```python
from build123d import *

# Parameters (mm, degrees)
F0_W        = 39
F0_H        = 39
F0_R        = 0.975
F1_DEPTH    = 9
F2_T1_DEPTH = 62
F4_DEPTH    = 21
F5_DEPTH    = 21
F6_DEPTH    = 5.5
F7_DEPTH    = 1.5
F8_DEPTH    = 2.5
F9_DEPTH    = 1.5
F10_R       = 1.25
F11_DEPTH   = 2.5
F12_DEPTH   = 5
F13_DEPTH   = 1


# Not quite as in the source:
# - a fillet or chamfer that OpenCascade refuses, or shapes differently, is made with other operations: its cross-section is extruded or revolved along the edge and cut away or added


with BuildPart() as f1:
    # F0 (on Top) → F1 (new body)
    with BuildSketch(Plane.XY):
        Polygon((-2.625, 21), (-21, 21), (-21, -21), (-2.625, -21), (2.625, -21), (21, -21), (21, 21), (2.625, 21), align=None)
        Rectangle(F0_W, F0_H, mode=Mode.SUBTRACT)
        Rectangle(F0_W, F0_H)
        with BuildLine():
            ThreePointArc((16, 4.25), (16.6, 4.85), (17.2, 4.25))
            Line((17.2, 4.25), (17.2, -4.25))
            ThreePointArc((17.2, -4.25), (16.6, -4.85), (16, -4.25))
            Line((16, -4.25), (16, -6.5))
            ThreePointArc((16, -6.5), (16.6, -5.9), (17.2, -6.5))
            Line((17.2, -6.5), (17.2, -15.7))
            ThreePointArc((17.2, -15.7), (18.2606601718, -18.2606601718), (15.7, -17.2))
            Line((15.7, -17.2), (6.5, -17.2))
            ThreePointArc((6.5, -17.2), (5.9, -16.6), (6.5, -16))
            Line((6.5, -16), (4.25, -16))
            ThreePointArc((4.25, -16), (4.85, -16.6), (4.25, -17.2))
            Line((4.25, -17.2), (-4.25, -17.2))
            ThreePointArc((-4.25, -17.2), (-4.85, -16.6), (-4.25, -16))
            Line((-4.25, -16), (-6.5, -16))
            ThreePointArc((-6.5, -16), (-5.9, -16.6), (-6.5, -17.2))
            Line((-6.5, -17.2), (-15.7, -17.2))
            ThreePointArc((-15.7, -17.2), (-18.2606601718, -18.2606601718), (-17.2, -15.7))
            Line((-17.2, -15.7), (-17.2, -6.5))
            ThreePointArc((-17.2, -6.5), (-16.6, -5.9), (-16, -6.5))
            Line((-16, -6.5), (-16, -4.25))
            ThreePointArc((-16, -4.25), (-16.6, -4.85), (-17.2, -4.25))
            Line((-17.2, -4.25), (-17.2, 4.25))
            ThreePointArc((-17.2, 4.25), (-16.6, 4.85), (-16, 4.25))
            Line((-16, 4.25), (-16, 6.5))
            ThreePointArc((-16, 6.5), (-16.6, 5.9), (-17.2, 6.5))
            Line((-17.2, 6.5), (-17.2, 15.7))
            ThreePointArc((-17.2, 15.7), (-18.2606601718, 18.2606601718), (-15.7, 17.2))
            Line((-15.7, 17.2), (-6.5, 17.2))
            ThreePointArc((-6.5, 17.2), (-5.9, 16.6), (-6.5, 16))
            Line((-6.5, 16), (-4.25, 16))
            ThreePointArc((-4.25, 16), (-4.85, 16.6), (-4.25, 17.2))
            Line((-4.25, 17.2), (4.25, 17.2))
            ThreePointArc((4.25, 17.2), (4.85, 16.6), (4.25, 16))
            Line((4.25, 16), (6.5, 16))
            ThreePointArc((6.5, 16), (5.9, 16.6), (6.5, 17.2))
            Line((6.5, 17.2), (15.7, 17.2))
            ThreePointArc((15.7, 17.2), (18.2606601718, 18.2606601718), (17.2, 15.7))
            Line((17.2, 15.7), (17.2, 6.5))
            ThreePointArc((17.2, 6.5), (16.6, 5.9), (16, 6.5))
            Line((16, 6.5), (16, 4.25))
        make_face(mode=Mode.SUBTRACT)
        Polygon((16, -4.25), (16, 4.25), (16, 6.5), (16, 16), (6.5, 16), (4.25, 16), (-4.25, 16), (-6.5, 16), (-16, 16), (-16, 6.5), (-16, 4.25), (-16, -4.25), (-16, -6.5), (-16, -16), (-6.5, -16), (-4.25, -16), (4.25, -16), (6.5, -16), (16, -16), (16, -6.5), align=None)
        with Locations((-14, -14)):
            Circle(F0_R, mode=Mode.SUBTRACT)
        with Locations((14, -14)):
            Circle(F0_R, mode=Mode.SUBTRACT)
        with Locations((-14, 14)):
            Circle(F0_R, mode=Mode.SUBTRACT)
        Polygon((-8.75, 14), (0, 14), (0, 10.75), (-8.75, 10.75), (-9.75, 10.75), (-9.75, 14), align=None, mode=Mode.SUBTRACT)
        with BuildLine():
            Line((-8.75, 8.75), (8.75, 8.75))
            Line((8.75, 8.75), (8.75, 2.75))
            Line((8.75, 2.75), (10.75, 2.75))
            ThreePointArc((10.75, 2.75), (13.5, 0), (10.75, -2.75))
            Line((10.75, -2.75), (8.75, -2.75))
            Line((8.75, -2.75), (8.75, -8.75))
            Line((8.75, -8.75), (-8.75, -8.75))
            Line((-8.75, -8.75), (-8.75, -2.75))
            Line((-8.75, -2.75), (-10.75, -2.75))
            ThreePointArc((-10.75, -2.75), (-13.5, 0), (-10.75, 2.75))
            Line((-10.75, 2.75), (-8.75, 2.75))
            Line((-8.75, 2.75), (-8.75, 8.75))
        make_face(mode=Mode.SUBTRACT)
        Polygon((10.75, 3.8126846775), (10.75, 8.75), (10.75, 9.75), (14, 9.75), (14, 8.75), (14, 3.8126846775), align=None, mode=Mode.SUBTRACT)
        with Locations((14, 14)):
            Circle(F0_R, mode=Mode.SUBTRACT)
        Polygon((0, 10.75), (0, 14), (-8.75, 14), (-9.75, 14), (-9.75, 10.75), (-8.75, 10.75), align=None)
        Polygon((10.75, 9.75), (10.75, 8.75), (10.75, 3.8126846775), (14, 3.8126846775), (14, 8.75), (14, 9.75), align=None)
        with Locations((14, -14)):
            Circle(F0_R)
        with Locations((-14, -14)):
            Circle(F0_R)
        with Locations((-14, 14)):
            Circle(F0_R)
        with Locations((14, 14)):
            Circle(F0_R)
    extrude(amount=F1_DEPTH)

    # F2: fillet of radius 4 on 2 edges, made by hand

    # F2_s2 → F2_t1 (cut)
    with BuildSketch(Plane.XZ.offset(-31)):
        with BuildLine():
            ThreePointArc((-21, 5), (-19.8284271247, 7.8284271247), (-17, 9))
            Line((-17, 9), (-21, 9))
            Line((-21, 9), (-21, 5))
        make_face()
        with BuildLine():
            ThreePointArc((21, 5), (19.8284271247, 7.8284271247), (17, 9))
            Line((17, 9), (21, 9))
            Line((21, 9), (21, 5))
        make_face()
    extrude(amount=F2_T1_DEPTH, mode=Mode.SUBTRACT)

    # F3 (on Right) → F4 (join)
    with BuildSketch(Plane.YZ):
        with BuildLine():
            Line((-21, 0), (-21, 1.1))
            ThreePointArc((-21, 1.1), (-21.875, 0.8183492931), (-22.75, 1.1))
            Line((-22.75, 1.1), (-22.75, 3.85))
            Line((-22.75, 3.85), (-24, 3.85))
            Line((-24, 3.85), (-26.75, 1.1))
            Line((-26.75, 1.1), (-26.75, -1.5))
            Line((-26.75, -1.5), (-22.75, -1.5))
            Line((-22.75, -1.5), (-21, -1.5))
            Line((-21, -1.5), (-21, 0))
        make_face()
    extrude(amount=F4_DEPTH)

    # F5 (add): a face of the model
    f5_faces = [f1.faces().sort_by_distance(p)[0] for p in [
        (0, -24.00739598, 0.5868334208),
    ]]
    extrude(f5_faces, amount=F5_DEPTH)

    # F0 (on Top) → F6 (join)
    with BuildSketch(Plane.XY):
        with Locations((-14, -14)):
            Circle(F0_R)
        with Locations((14, -14)):
            Circle(F0_R)
        with Locations((-14, 14)):
            Circle(F0_R)
        with Locations((14, 14)):
            Circle(F0_R)
    extrude(amount=-F6_DEPTH)

    # F0 (on Top) → F7 (join)
    with BuildSketch(Plane.XY):
        Rectangle(F0_W, F0_H)
        with BuildLine():
            ThreePointArc((16, 4.25), (16.6, 4.85), (17.2, 4.25))
            Line((17.2, 4.25), (17.2, -4.25))
            ThreePointArc((17.2, -4.25), (16.6, -4.85), (16, -4.25))
            Line((16, -4.25), (16, -6.5))
            ThreePointArc((16, -6.5), (16.6, -5.9), (17.2, -6.5))
            Line((17.2, -6.5), (17.2, -15.7))
            ThreePointArc((17.2, -15.7), (18.2606601718, -18.2606601718), (15.7, -17.2))
            Line((15.7, -17.2), (6.5, -17.2))
            ThreePointArc((6.5, -17.2), (5.9, -16.6), (6.5, -16))
            Line((6.5, -16), (4.25, -16))
            ThreePointArc((4.25, -16), (4.85, -16.6), (4.25, -17.2))
            Line((4.25, -17.2), (-4.25, -17.2))
            ThreePointArc((-4.25, -17.2), (-4.85, -16.6), (-4.25, -16))
            Line((-4.25, -16), (-6.5, -16))
            ThreePointArc((-6.5, -16), (-5.9, -16.6), (-6.5, -17.2))
            Line((-6.5, -17.2), (-15.7, -17.2))
            ThreePointArc((-15.7, -17.2), (-18.2606601718, -18.2606601718), (-17.2, -15.7))
            Line((-17.2, -15.7), (-17.2, -6.5))
            ThreePointArc((-17.2, -6.5), (-16.6, -5.9), (-16, -6.5))
            Line((-16, -6.5), (-16, -4.25))
            ThreePointArc((-16, -4.25), (-16.6, -4.85), (-17.2, -4.25))
            Line((-17.2, -4.25), (-17.2, 4.25))
            ThreePointArc((-17.2, 4.25), (-16.6, 4.85), (-16, 4.25))
            Line((-16, 4.25), (-16, 6.5))
            ThreePointArc((-16, 6.5), (-16.6, 5.9), (-17.2, 6.5))
            Line((-17.2, 6.5), (-17.2, 15.7))
            ThreePointArc((-17.2, 15.7), (-18.2606601718, 18.2606601718), (-15.7, 17.2))
            Line((-15.7, 17.2), (-6.5, 17.2))
            ThreePointArc((-6.5, 17.2), (-5.9, 16.6), (-6.5, 16))
            Line((-6.5, 16), (-4.25, 16))
            ThreePointArc((-4.25, 16), (-4.85, 16.6), (-4.25, 17.2))
            Line((-4.25, 17.2), (4.25, 17.2))
            ThreePointArc((4.25, 17.2), (4.85, 16.6), (4.25, 16))
            Line((4.25, 16), (6.5, 16))
            ThreePointArc((6.5, 16), (5.9, 16.6), (6.5, 17.2))
            Line((6.5, 17.2), (15.7, 17.2))
            ThreePointArc((15.7, 17.2), (18.2606601718, 18.2606601718), (17.2, 15.7))
            Line((17.2, 15.7), (17.2, 6.5))
            ThreePointArc((17.2, 6.5), (16.6, 5.9), (16, 6.5))
            Line((16, 6.5), (16, 4.25))
        make_face(mode=Mode.SUBTRACT)
    extrude(amount=-F7_DEPTH)

    # F8 (cut): a face of the model
    f8_faces = [f1.faces().sort_by_distance(p)[0] for p in [
        (-18.9484567107, 0, -1.5),
    ]]
    extrude(f8_faces, amount=-F8_DEPTH, mode=Mode.SUBTRACT)

    # F0 (on Top) → F9 (join)
    with BuildSketch(Plane.XY):
        Polygon((-2.625, 21), (-21, 21), (-21, -21), (-2.625, -21), (2.625, -21), (21, -21), (21, 21), (2.625, 21), align=None)
        Rectangle(F0_W, F0_H, mode=Mode.SUBTRACT)
    extrude(amount=-F9_DEPTH)

    # F10 (on face) → F11 (cut)
    with BuildSketch(Plane(origin=(0, 0, -1.5), x_dir=(1, 0, 0), z_dir=(0, 0, -1))):
        with Locations((10.5, 24.25)):
            Circle(F10_R)
        with Locations((0, 24.25)):
            Circle(F10_R)
        with Locations((-10.5, 24.25)):
            Circle(F10_R)
    extrude(amount=-F11_DEPTH, mode=Mode.SUBTRACT)

    # F0 (on Top) → F12 (cut)
    with BuildSketch(Plane.XY):
        Polygon((10.75, 9.75), (10.75, 8.75), (10.75, 3.8126846775), (14, 3.8126846775), (14, 8.75), (14, 9.75), align=None)
        Polygon((0, 10.75), (0, 14), (-8.75, 14), (-9.75, 14), (-9.75, 10.75), (-8.75, 10.75), align=None)
    extrude(amount=F12_DEPTH, mode=Mode.SUBTRACT)

    # F0 (on Top) → F13 (cut)
    with BuildSketch(Plane.XY):
        Polygon((16, -4.25), (16, 4.25), (16, 6.5), (16, 16), (6.5, 16), (4.25, 16), (-4.25, 16), (-6.5, 16), (-16, 16), (-16, 6.5), (-16, 4.25), (-16, -4.25), (-16, -6.5), (-16, -16), (-6.5, -16), (-4.25, -16), (4.25, -16), (6.5, -16), (16, -16), (16, -6.5), align=None)
        with Locations((-14, -14)):
            Circle(F0_R, mode=Mode.SUBTRACT)
        with Locations((14, -14)):
            Circle(F0_R, mode=Mode.SUBTRACT)
        with Locations((-14, 14)):
            Circle(F0_R, mode=Mode.SUBTRACT)
        Polygon((-8.75, 14), (0, 14), (0, 10.75), (-8.75, 10.75), (-9.75, 10.75), (-9.75, 14), align=None, mode=Mode.SUBTRACT)
        with BuildLine():
            Line((-8.75, 8.75), (8.75, 8.75))
            Line((8.75, 8.75), (8.75, 2.75))
            Line((8.75, 2.75), (10.75, 2.75))
            ThreePointArc((10.75, 2.75), (13.5, 0), (10.75, -2.75))
            Line((10.75, -2.75), (8.75, -2.75))
            Line((8.75, -2.75), (8.75, -8.75))
            Line((8.75, -8.75), (-8.75, -8.75))
            Line((-8.75, -8.75), (-8.75, -2.75))
            Line((-8.75, -2.75), (-10.75, -2.75))
            ThreePointArc((-10.75, -2.75), (-13.5, 0), (-10.75, 2.75))
            Line((-10.75, 2.75), (-8.75, 2.75))
            Line((-8.75, 2.75), (-8.75, 8.75))
        make_face(mode=Mode.SUBTRACT)
        Polygon((10.75, 3.8126846775), (10.75, 8.75), (10.75, 9.75), (14, 9.75), (14, 8.75), (14, 3.8126846775), align=None, mode=Mode.SUBTRACT)
        with Locations((14, 14)):
            Circle(F0_R, mode=Mode.SUBTRACT)
    extrude(amount=F13_DEPTH, mode=Mode.SUBTRACT)


solid = f1.part
```
Part model, mm, in its own coordinate system. A direction names the side the tool comes from. Round coordinates to 2 decimals unless told otherwise and drop trailing zeros. Loops run counter-clockwise (first coordinate to the right, second up) from the corner with the lowest first, then second, coordinate; pieces in that order, holes last. Notation, with made-up numbers: (35.25, -10) -> (54.25, -10) arc R19 ccw to (54.25, 12) -> close; hole circle Ø9 at (-34, 5). An arc over 180 degrees is marked (long way). Use one line per item in the form item = value. Start each with the question number.
Item 1: Drop flat-ended pins along their axis: pin 1 Ø4 at (x, y) = (2, -15) entering from -Z; pin 2 Ø6.5 at (x, z) = (-4, 4.5) entering from -Y; pin 3 Ø6 at (x, z) = (11.5, 2) entering from -Y; pin 4 Ø2.5 at (y, z) = (-1, 6.5) entering from -X. Give the stop position or say it passes through.
Item 2: Band-saw the part on D-D (y = 1). List the corners of the cut face in (x, z) (3 decimals), plus the area to 3 significant figures.
Item 3: Tool access for faces 1 (the flat face through (0, 12, 3)), 2 (the flat face through (-14, 14, -5.5)), 3 (the flat face through (17.2, 11, 5)): list every direction of +Z, -Z, +X, -X, +Y, -Y with a clear straight run to the whole face (end or side of a thin tool).
Item 4: Drill centre lines: line 1 along X through (y, z) = (-24.25, -0.45); line 2 along X through (y, z) = (9.5, 4.5); line 3 along X through (y, z) = (3.5, 0.5). Where is each one in solid material? Low to high.
Item 5: Two-plate mould, pull along X, no slides. Class faces 4 (the flat face through (-9.75, 12, 3)), 5 (the flat face through (0, -22.75, 2)): released by +X, released by -X, zero draft, split by the parting line, or undercut.
Item 6: Band-saw the part on C-C (x = 18). List the corners of the cut face in (y, z) (3 decimals).
Item 7: Band-saw the part on A-A (y = -12). List the corners of the cut face in (x, z) (3 decimals).
Item 8: Band-saw the part on B-B (z = -2.5). List the corners of the cut face in (x, y) (3 decimals).
Data:
q1.pin_1 = 1
q1.pin_2 = -26.6
q1.pin_3 = -26.75
q1.pin_4 = -20.99
q2.outline = (-21, -1.5) -> (-19.5, -1.5) -> (-19.5, 1) -> (-17.2, 1) -> (-17.2, 8.995) arc R4 ccw to (-21, 5) -> close; (-16, 1) -> (-13.312, 1) -> (-13.312, 9) -> (-16, 9) -> close; (13.312, 1) -> (16, 1) -> (16, 9) -> (13.312, 9) -> close; (17.2, 1) -> (19.5, 1) -> (19.5, -1.5) -> (21, -1.5) -> (21, 5) arc R4 ccw to (17.2, 8.995) -> close
q2.area = 104 mm^2
q3.face_1 = -Z
q3.face_2 = -Z, +X, -X, +Y, -Y
q3.face_3 = +Z, -Z
q4.line_1 = -21 to -11.75, -9.25 to -1.25, 1.25 to 9.25, 11.75 to 21
q4.line_2 = -21 to -17.2, -16 to 10.75, 14 to 16, 17.2 to 21
q4.line_3 = -21 to -19.5, 19.5 to 21
q5.face_4 = undercut
q5.face_5 = zero draft
q6.outline = (-26.75, -1.5) -> (-19.5, -1.5) -> (-19.5, 1) -> (-18.469, 1) -> (-18.469, 8.873) -> (-21, 8.873) -> (-21, 1.1) arc R1.5 cw to (-22.75, 1.1) -> (-22.75, 3.85) -> (-24, 3.85) -> (-26.75, 1.1) -> close; (-15.931, 1) -> (15.931, 1) -> (15.931, 8.873) -> (-15.931, 8.873) -> close; (18.469, 1) -> (19.5, 1) -> (19.5, -1.5) -> (21, -1.5) -> (21, 8.873) -> (18.469, 8.873) -> close
q7.outline = (-21, -1.5) -> (-19.5, -1.5) -> (-19.5, 1) -> (-17.2, 1) -> (-17.2, 8.995) arc R4 ccw to (-21, 5) -> close; (-16, 1) -> (16, 1) -> (16, 9) -> (-16, 9) -> close; (17.2, 1) -> (19.5, 1) -> (19.5, -1.5) -> (21, -1.5) -> (21, 5) arc R4 ccw to (17.2, 8.995) -> close
q8.outline = circle Ø1.95 at (-14, -14); circle Ø1.95 at (-14, 14); circle Ø1.95 at (14, -14); circle Ø1.95 at (14, 14)
